Geometry: see drawing. Coordinates: mm, zero at the bounding-box minimum. A direction names the side the tool comes from. Round coordinates to 2 decimals unless told otherwise and drop trailing zeros. Write each loop counter-clockwise with the first axis right and the second up, starting at its lowest first coordinate (ties: lowest second). Pieces come first, ordered by that corner, then holes.
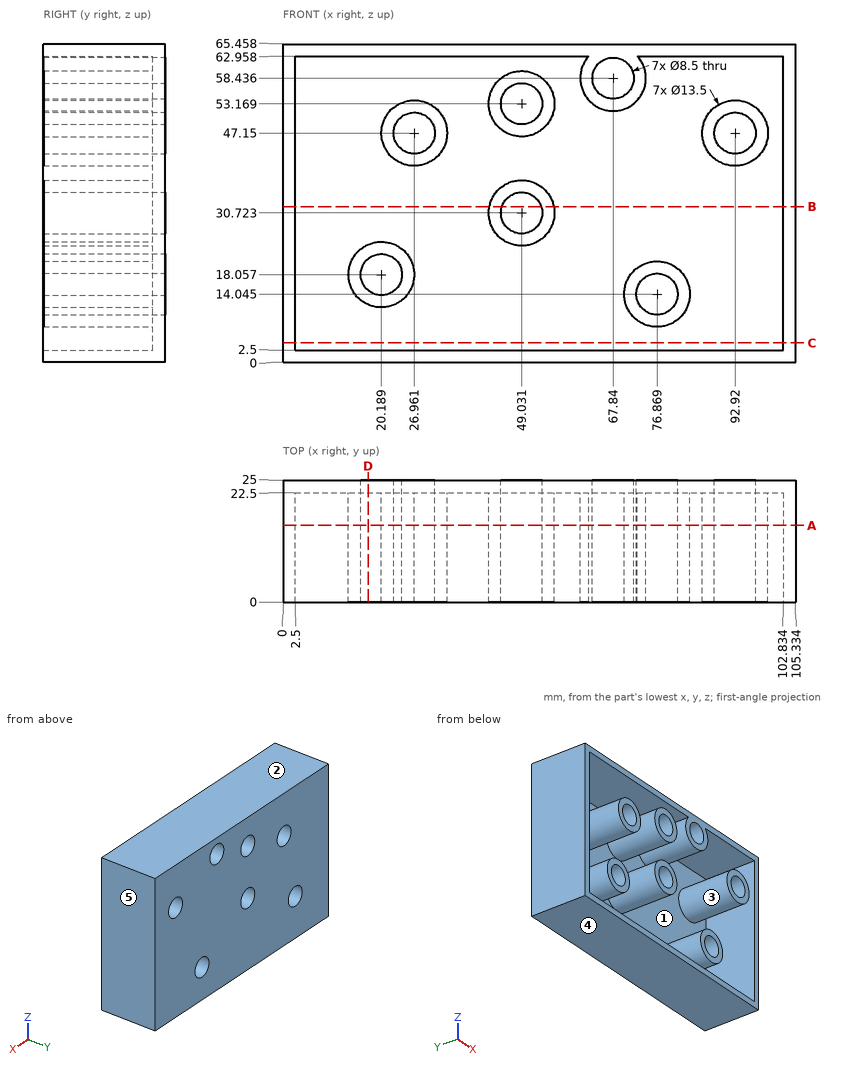
1) Section query B-B on z = 32. Return the cut outline in (x, y) (1 decimal).
Taken from the geometry:
outline: (0, 0) - (2.5, 0) - (2.5, 22.5) - (42.4, 22.5) - (42.4, 0) - (45, 0) - (45, 25) - (0, 25) - close; (53.1, 0) - (55.7, 0) - (55.7, 22.5) - (102.8, 22.5) - (102.8, 0) - (105.3, 0) - (105.3, 25) - (53.1, 25) - close
2) Contact query for flat-ended pins moving along their axis: P1, Ø8, axis at x = 42, z = 41, coming from the -Y side; P2, Ø5, axis at x = 92.92, z = 47.15, coming from the +Y side. Output: stop coordinate, or through.
Taken from the geometry:
P1: stops at y = 22.5
P2: passes through
3) Reachability of the marked faces 1 and 2 from +Z, -Z, +X, -X, +Y, -Y: full face, straight path, thin tool, end or side. Return the list, or none.
Taken from the geometry:
face 1: -Y
face 2: +Z, +X, -X, +Y, -Y
4) Section query A-A on y = 15.75. State how many separate pieces and enclosed holes the cut face has, then the cut area to 3 significant figures.
Taken from the geometry:
separate pieces: 7
enclosed holes: 8
area: 1,420 mm2
5) Pull-direction query (Z, two-part tool) for the marked faces 3, 4 and 5; classes: released by +Z, released by -Z, zero draft, split by the parting line, or undercut.
Taken from the geometry:
face 3: undercut
face 4: released by -Z
face 5: zero draft
6) Material intervals for line 1 (Z direction, x = 27, y = 11); line 2 (Z direction, x = 9, y = 14); line 3 (Z direction, x = 68.5, y = 5.5) (1 decimal), sorted ascending.
Taken from the geometry:
line 1: z = 0 to 2.5, 40.4 to 42.9, 51.4 to 53.9, 62.96 to 65.46
line 2: z = 0 to 2.5, 62.96 to 65.46
line 3: z = 0 to 2.5, 51.7 to 54.2, 62.6 to 65.5
7) Section query C-C on z = 4. Return the cut outline in (x, y) (1 decimal).
Taken from the geometry:
outline: (0, 0) - (2.5, 0) - (2.5, 22.5) - (102.8, 22.5) - (102.8, 0) - (105.3, 0) - (105.3, 25) - (0, 25) - close
8) Section query D-D on x = 17.5. Return the cut outline in (y, z), then the cut area to 3 significant figures.
Taken from the geometry:
outline: (0, 0) - (25, 0) - (25, 14.77) - (0, 14.77) - (0, 11.87) - (22.5, 11.87) - (22.5, 2.5) - (0, 2.5) - close; (0, 21.35) - (25, 21.35) - (25, 65.46) - (0, 65.46) - (0, 62.96) - (22.5, 62.96) - (22.5, 24.25) - (0, 24.25) - close
area: 390 mm2
